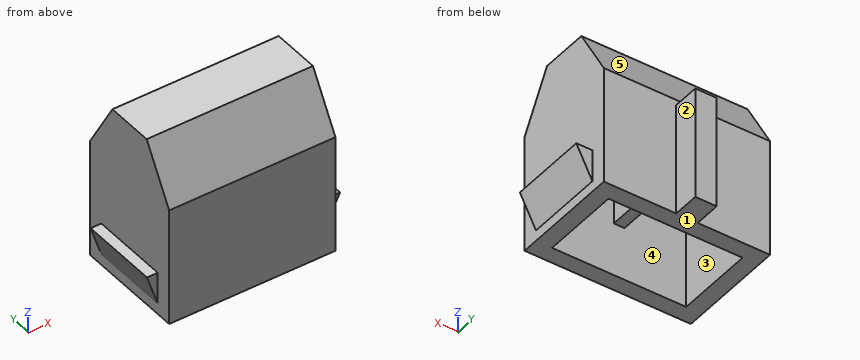
Autodesk Fusion 360 part; units mm, degrees
sketch "Rail Sketch" plane through (0, 0, 0) normal (1, 0, 0) x (0, 0, -1)
  line L0 (0, 0) -> (0, 10.4)
  line L1 (0, 10.4) -> (-11, 10.4)
  line L2 (-11, 0) -> (-16, 2.95)
  line L3 (-16, 7.45) -> (-11, 10.4)
  line L4 (-16, 2.95) -> (-16, 7.45)
  line L5 (-11, 0) -> (0, 0)
  dimension "d1" = 5
  dimension "d2" = 4.5
  dimension "d3" = 10.4
  dimension "d4" = 16
extrude "Extrude1" add sketch "Rail Sketch" along normal blind 15.5
sketch "Back Hole" plane through (0, 0, 0) normal (0, 0, -1) x (-1, 0, 0)
  line L0 (0, 0) -> (0, 10.4)
  line L1 (0, 10.4) -> (-15.5, 10.4)
  line L2 (-15.5, 10.4) -> (-15.5, 0)
  line L3 (-15.5, 0) -> (0, 0)
  line L4 (-14, 8.9) -> (-1.5, 8.9)
  line L5 (-1.5, 8.9) -> (-1.5, 1.5)
  line L6 (-1.5, 1.5) -> (-14, 1.5)
  line L7 (-14, 1.5) -> (-14, 8.9)
  dimension "d8" = 1.5
  dimension "d9" = 1.5
  dimension "d10" = 1.5
  dimension "d11" = 1.5
extrude "Extrude2" cut sketch "Back Hole" against normal blind 11.5 contours L4 L5 L6 L7
sketch "Cross" plane through (0, 0, 11.5) normal (0, 0, -1) x (-1, 0, 0)
  line L0 (-14, 1.5) -> (-1.5, 1.5)
  line L1 (-1.5, 1.5) -> (-1.5, 8.9)
  line L2 (-1.5, 8.9) -> (-14, 8.9)
  line L3 (-14, 8.9) -> (-14, 1.5)
  line L4 (-7.75, 8.9) -> (-8.25, 8.9)
  line L5 (-8.25, 5.7) -> (-14, 5.7)
  line L6 (-14, 5.2) -> (-14, 4.7)
  line L7 (-8.25, 4.7) -> (-8.25, 1.5)
  line L8 (-7.75, 1.5) -> (-7.25, 1.5)
  line L9 (-7.25, 4.7) -> (-1.5, 4.7)
  line L10 (-1.5, 5.2) -> (-1.5, 5.7)
  line L11 (-14, 4.7) -> (-8.25, 4.7)
  line L12 (-7.25, 1.5) -> (-7.25, 1.6)
  line L13 (-7.25, 1.6) -> (-7.25, 4.7)
  line L14 (-1.5, 4.7) -> (-1.5, 5.2)
  line L15 (-1.5, 5.7) -> (-7.25, 5.7)
  line L16 (-7.25, 5.7) -> (-7.25, 8.9)
  line L17 (-7.75, 8.9) -> (-7.25, 8.9)
  line L18 (-8.25, 8.9) -> (-8.25, 5.7)
  line L19 (-8.25, 1.5) -> (-7.75, 1.5)
  line L20 (-14, 5.7) -> (-14, 5.2)
  dimension "d16" = 1
extrude "Extrude3" add sketch "Cross" along normal blind 6.5 contours L0 L1 L2 L3 L4 L5 L6 L7 L8 L9 L10 L11 L12 L13 L14 L15 L16 L17 L18 L19 L20
sketch "Vertical Support" plane through (0, 0, 0) normal (0, 0, -1) x (-1, 0, 0)
  line L0 (-1.5, 8.9) -> (-1.5, 1.5)
  line L1 (-1.5, 1.5) -> (-14, 1.5)
  line L2 (-14, 1.5) -> (-14, 8.9)
  line L3 (-14, 8.9) -> (-1.5, 8.9)
  line L4 (0, 0) -> (0, 10.4)
  line L5 (0, 10.4) -> (-15.5, 10.4)
  line L6 (-15.5, 10.4) -> (-15.5, 0)
  line L7 (-15.5, 0) -> (0, 0)
  line L8 (-8.75, 10.4) -> (-7.75, 10.4)
  line L9 (-7.75, 10.4) -> (-6.75, 10.4)
  line L10 (-6.75, 12.9) -> (-6.75, 10.4)
  line L11 (-6.75, 12.9) -> (-8.75, 12.9)
  line L12 (-8.75, 12.9) -> (-8.75, 10.4)
  dimension "d19" = 2
  dimension "d20" = 2.5
extrude "Extrude4" add sketch "Vertical Support" against normal blind 10.5 contours L5 L8 L9 L10 L11 L12
sketch "Right Fin " plane through (15.5, 0, 0) normal (1, 0, 0) x (0, 0, -1)
  line L0 (-16, 2.95) -> (-11, 0)
  line L1 (-11, 0) -> (0, 0)
  line L2 (0, 0) -> (0, 10.4)
  line L3 (0, 10.4) -> (-11, 10.4)
  line L4 (-11, 10.4) -> (-16, 7.45)
  line L5 (-16, 7.45) -> (-16, 2.95)
  line L6 (-1, 8.9) -> (-1, 1.5)
  line L7 (-1, 1.5) -> (-4, 1.5)
  line L8 (-4, 1.5) -> (-4, 8.9)
  line L9 (-4, 8.9) -> (-1, 8.9)
  dimension "d23" = 1.5
  dimension "d24" = 1.5
  dimension "d25" = 3
  dimension "d26" = 1
extrude "Extrude5" add sketch "Right Fin " along normal blind 1.5 contours L6 L7 L8 L9
sketch "Right Fin Slice" plane through (0, 8.9, 0) normal (0, 1, 0) x (-1, 0, 0)
  line L0 (-15.5, 1) -> (-15.5, 4)
  line L1 (-15.5, 4) -> (-17, 4)
  line L2 (-17, 4) -> (-17, 1)
  line L3 (-17, 1) -> (-15.5, 1)
  line L4 (-15.5, 1) -> (-17, 4)
extrude "Extrude6" cut sketch "Right Fin Slice" against normal blind 7.4 contours L2 L3 L4
sketch "Left Fin" plane through (0, 0, 0) normal (-1, 0, 0) x (0, 0, 1)
  line L0 (11, 0) -> (16, 2.95)
  line L1 (16, 2.95) -> (16, 7.45)
  line L2 (16, 7.45) -> (11, 10.4)
  line L3 (11, 10.4) -> (0, 10.4)
  line L4 (0, 10.4) -> (0, 0)
  line L5 (0, 0) -> (11, 0)
  line L6 (1, 8.9) -> (4, 8.9)
  line L7 (4, 8.9) -> (4, 1.5)
  line L8 (4, 1.5) -> (1, 1.5)
  line L9 (1, 1.5) -> (1, 8.9)
  dimension "d31" = 1
  dimension "d32" = 3
  dimension "d33" = 1.5
  dimension "d34" = 1.5
extrude "Extrude7" add sketch "Left Fin" along normal blind 1 contours L6 L7 L8 L9
sketch "Left Fin Slice" plane through (0, 8.9, 0) normal (0, 1, 0) x (-1, 0, 0)
  line L0 (0, 4) -> (0, 1)
  line L1 (0, 1) -> (1, 1)
  line L2 (1, 1) -> (1, 4)
  line L3 (1, 4) -> (0, 4)
  line L4 (0, 1) -> (1, 4)
extrude "Extrude8" cut sketch "Left Fin Slice" against normal blind 7.4 contours L1 L2 L4
equation "d17 = 11.5 mm - 5 mm"
Build history of the part. All positions in model axes, mm. Face numbers are marked on the shaded views. A direction names the side the tool comes from. Give positions to 0.01 mm unless a question says otherwise; leave off trailing zeros. Loops run counter-clockwise (first coordinate to the right, second up) from the corner with the lowest first, then second, coordinate; pieces in that order, holes last.
Item 1: Pull direction X, two halves, no side cores. Call the marked faces 1, 2 and 3: released by +X, released by -X, zero draft, split by the parting line, or undercut.
Answers follow:
face 1: zero draft
face 2: released by +X
face 3: undercut
Item 2: Slice it at A-A, the plane z = 4.75. List the corners of the cut face in (x, y).
Answers follow:
outline: (0, 0) - (15.5, 0) - (15.5, 10.4) - (8.75, 10.4) - (8.75, 12.9) - (6.75, 12.9) - (6.75, 10.4) - (0, 10.4) - close; hole (1.5, 1.5) - (14, 1.5) - (14, 8.9) - (1.5, 8.9) - close
Item 3: Slice it at B-B, the plane y = 6. List the corners of the cut face in (x, z), and give its area (4 significant figures).
Answers follow:
outline: (-1, 4) - (0, 1) - (0, 0) - (1.5, 0) - (1.5, 11.5) - (7.25, 11.5) - (7.25, 5) - (8.25, 5) - (8.25, 11.5) - (14, 11.5) - (14, 0) - (15.5, 0) - (15.5, 1) - (17, 4) - (15.5, 4) - (15.5, 16) - (0, 16) - (0, 4) - close
area: 114.5 mm2
Item 4: Which spindle directions (+Z, -Z, +X, -X, +Y, -Y) get a long thin tool onto all of the face, cutting with end or side? Do the marked faces 4 and 5. Say none if no direction does.
Answers follow:
face 4: -Z
face 5: +Z, +X, -X, +Y
Item 5: Drill centre lines: line 1 (X direction, y = 3.5, z = 10.5); line 2 (Y direction, x = 3, z = 9.25); line 3 (Y direction, x = 6.5, z = 3.75). Where is each one in solid material? Low to high.
Answers follow:
line 1: x = 0 to 1.5, 7.25 to 8.25, 14 to 15.5
line 2: y = 0 to 1.5, 4.7 to 5.7, 8.9 to 10.4
line 3: y = 0 to 1.5, 8.9 to 10.4
Item 6: Slice it at C-C, the plane x = 8. List the corners of the cut face in (y, z), and give its area (3 significant figures).
Answers follow:
outline: (0, 0) - (1.5, 0) - (1.5, 5) - (8.9, 5) - (8.9, 0) - (12.9, 0) - (12.9, 10.5) - (10.4, 10.5) - (10.4, 11) - (7.45, 16) - (2.95, 16) - (0, 11) - close
area: 141 mm2
Item 7: Flat gauge pins, fed straight in: pin 1 (2 mm diameter, centred on x = 9.5, y = 5, fed in from -Z); pin 2 (1.7 mm diameter, centred on x = 10, z = 7.5, fed in from +Y); pin 3 (0.8 mm diameter, centred on y = 12, z = 7, fed in from +X); pin 4 (6 mm diameter, centred on x = 12.5, y = 5, fed in from -Z). Where does each tip first touch, or does it go through?
Answers follow:
pin 1: stops at z = 5
pin 2: stops at y = 10.4
pin 3: stops at x = 8.75
pin 4: stops at z = 0
Item 8: Slice it at D-D, the plane z = 2.5. List the corners of the cut face in (x, y).
Answers follow:
outline: (-0.5, 1.5) - (0, 1.5) - (0, 0) - (15.5, 0) - (15.5, 1.5) - (16.25, 1.5) - (16.25, 8.9) - (15.5, 8.9) - (15.5, 10.4) - (8.75, 10.4) - (8.75, 12.9) - (6.75, 12.9) - (6.75, 10.4) - (0, 10.4) - (0, 8.9) - (-0.5, 8.9) - close; hole (1.5, 1.5) - (14, 1.5) - (14, 8.9) - (1.5, 8.9) - close
